Input: part model. Units: mm. Frame: model coordinates. Give positions to 0.01 mm unless a question says otherwise; leave off trailing zeros. Loops run counter-clockwise (first coordinate to the right, second up) from the corner with the lowest first, then second, coordinate; pieces in that order, holes last. Notation, with made-up numbers: (49, 65.5) -> (59, 65.5) arc R27 ccw to (59, 86.5) -> close; hole circle Ø9 at (55, 30.25). An arc over 180 degrees is marked (long way). Answer as a JSON object with one key per item and string values.
```python
from build123d import *

# Parameters (mm, degrees)
BOSS_EXTRUDE1_DEPTH = 6.35
SKETCH2_R           = 4.7625
CUT_EXTRUDE1_DEPTH  = 7.35
CHAMFER2_SIZE       = 0.254
CHAMFER2_SIZE2      = 0.022222121
CHAMFER3_SIZE       = 0.254
CHAMFER3_SIZE2      = 0.022222121
SKETCH3_OUTSIDE_W   = 33.55
SKETCH3_OUTSIDE_H   = 35.762
SKETCH3_OUTSIDE_R   = 7.150103868
CUT_EXTRUDE2_DEPTH  = 6.35
CUT_EXTRUDE2_TAPER  = 45
SKETCH4_OUTSIDE_W   = 33.55
SKETCH4_OUTSIDE_H   = 35.762
SKETCH4_OUTSIDE_R   = 7.1501
CUT_EXTRUDE3_DEPTH  = 6.35
CUT_EXTRUDE3_TAPER  = 45


with BuildPart() as part:
    # Sketch1 → Boss-Extrude1 (new body)
    with BuildSketch(Plane(origin=(0, 0, 0), x_dir=(1, 0, 0), z_dir=(0, 1, 0))):
        Polygon((0, 8.256224319), (-7.1501, 4.12811216), (-7.1501, -4.12811216), (0, -8.256224319), (7.1501, -4.12811216), (7.1501, 4.12811216), align=None)
    extrude(amount=BOSS_EXTRUDE1_DEPTH)

    # Sketch2 → Cut-Extrude1 (cut, through all)
    with BuildSketch(Plane(origin=(0, 6.35, 0), x_dir=(1, 0, 0), z_dir=(0, 1, 0))):
        Circle(SKETCH2_R)
    extrude(amount=-CUT_EXTRUDE1_DEPTH, mode=Mode.SUBTRACT)

    # Chamfer2
    chamfer2_edges = [part.edges().sort_by_distance(p)[0] for p in [
        (-4.7625, 6.35, 0),
    ]]
    chamfer2_side = [part.faces().sort_by_distance(p)[0] for p in [
        (-3.465830418, 6.35, -6.002994375),
    ]]
    chamfer(chamfer2_edges, length=CHAMFER2_SIZE, length2=CHAMFER2_SIZE2, reference=chamfer2_side[0])

    # Chamfer3
    chamfer3_edges = [part.edges().sort_by_distance(p)[0] for p in [
        (-4.7625, 0, 0),
    ]]
    chamfer3_side = [part.faces().sort_by_distance(p)[0] for p in [
        (-4.7625, 3.16388894, 0),
    ]]
    chamfer(chamfer3_edges, length=CHAMFER3_SIZE, length2=CHAMFER3_SIZE2, reference=chamfer3_side[0])

    # Sketch3 outside → Cut-Extrude2 (cut)
    with BuildSketch(Plane(origin=(0, 6.35, 0), x_dir=(1, 0, 0), z_dir=(0, 1, 0))):
        Rectangle(SKETCH3_OUTSIDE_W, SKETCH3_OUTSIDE_H)
        Circle(SKETCH3_OUTSIDE_R, mode=Mode.SUBTRACT)
    extrude(amount=-CUT_EXTRUDE2_DEPTH, taper=CUT_EXTRUDE2_TAPER, mode=Mode.SUBTRACT)

    # Sketch4 outside → Cut-Extrude3 (cut)
    with BuildSketch(Plane.XZ):
        Rectangle(SKETCH4_OUTSIDE_W, SKETCH4_OUTSIDE_H)
        Circle(SKETCH4_OUTSIDE_R, mode=Mode.SUBTRACT)
    extrude(amount=-CUT_EXTRUDE3_DEPTH, taper=CUT_EXTRUDE3_TAPER, mode=Mode.SUBTRACT)


solid = part.part
```
Q1. Draft query along X for faces 1 (the conical face through (6.416, 0.269, 3.725)), 2 (the conical face through (-6.4, 6.12, -3.67)), 3 (the cylindrical face through (-3.78, 3.33, 2.9)), 4 (the flat face through (1, 0, 5)). Return one class per face: +X half, -X half, draft (parallel to the pull), parting line (faces both ways), or undercut.
Evaluation:
{"face 1": "+X half", "face 2": "-X half", "face 3": "undercut", "face 4": "draft"}
Q2. Section A-A, the plane y = 5. Return the cut outline in (x, z) (1 decimal).
Evaluation:
{"outline": "(-7.2, -4.1) -> (0, -8.3) -> (7.2, -4.1) -> (7.2, 4.1) -> (0, 8.3) -> (-7.2, 4.1) -> close; hole circle Ø9.5 at (0, 0)"}
Q3. Pin query (flat end, axial travel): pin 1 (3 mm diameter, centred on y = 0.5, z = 6.5, fed in from -X). Return the tip coordinate at first contact, or that it passes through.
Evaluation:
{"pin 1": "stops at x = -5.64"}
Q4. Ray query, line 1 along X through (y, z) = (2.5, 0); line 2 along X through (y, z) = (6, 3.75); line 3 along Z through (x, y) = (-2, 5). Return the intervals inside material, ascending.
Evaluation:
{"line 1": "x = -7.15 to -4.76, 4.76 to 7.15", "line 2": "x = -6.5 to -2.94, 2.94 to 6.5", "line 3": "z = -7.1 to -4.32, 4.32 to 7.1"}
